```python
from build123d import *

# Parameters (mm, degrees)
F1_DEPTH = 200
F2_R     = 2
F3_DEPTH = 7.301
F6_DEPTH = 25
F9_DEPTH = 150


# Not quite as in the source:
# - a feature names something its author has since deleted; it is built from what else it names


with BuildPart() as f1:
    # F0 (on Front) → F1 (new body)
    with BuildSketch(Plane.XZ):
        with BuildLine():
            Line((7.0581561667, 0.685534298), (6.15, 1.65))
            ThreePointArc((6.15, 1.65), (5.5642135624, 3.0642135624), (4.15, 3.65))
            Line((4.15, 3.65), (-4.15, 3.65))
            ThreePointArc((-4.15, 3.65), (-5.5642135624, 3.0642135624), (-6.15, 1.65))
            Line((-6.15, 1.65), (-7.0581561667, 0.685534298))
            ThreePointArc((-7.0581561667, 0.685534298), (-7.3301158338, 0), (-7.0581561667, -0.685534298))
            Line((-7.0581561667, -0.685534298), (-6.15, -1.65))
            ThreePointArc((-6.15, -1.65), (-5.5642135624, -3.0642135624), (-4.15, -3.65))
            Line((-4.15, -3.65), (4.15, -3.65))
            ThreePointArc((4.15, -3.65), (5.5642135624, -3.0642135624), (6.15, -1.65))
            Line((6.15, -1.65), (7.0581561667, -0.685534298))
            ThreePointArc((7.0581561667, -0.685534298), (7.3301158338, 0), (7.0581561667, 0.685534298))
        make_face()
        with BuildLine():
            ThreePointArc((5.15, -1.65), (4.8571067812, -2.3571067812), (4.15, -2.65))
            Line((4.15, -2.65), (-4.15, -2.65))
            ThreePointArc((-4.15, -2.65), (-4.8571067812, -2.3571067812), (-5.15, -1.65))
            Line((-5.15, -1.65), (-5.15, 1.65))
            ThreePointArc((-5.15, 1.65), (-4.8571067812, 2.3571067812), (-4.15, 2.65))
            Line((-4.15, 2.65), (4.15, 2.65))
            ThreePointArc((4.15, 2.65), (4.8571067812, 2.3571067812), (5.15, 1.65))
            Line((5.15, 1.65), (5.15, -1.65))
        make_face(mode=Mode.SUBTRACT)
        with BuildLine():
            Line((-4.15, -2.65), (4.15, -2.65))
            ThreePointArc((4.15, -2.65), (4.8571067812, -2.3571067812), (5.15, -1.65))
            Line((5.15, -1.65), (5.15, 1.65))
            ThreePointArc((5.15, 1.65), (4.8571067812, 2.3571067812), (4.15, 2.65))
            Line((4.15, 2.65), (-4.15, 2.65))
            ThreePointArc((-4.15, 2.65), (-4.8571067812, 2.3571067812), (-5.15, 1.65))
            Line((-5.15, 1.65), (-5.15, -1.65))
            ThreePointArc((-5.15, -1.65), (-4.8571067812, -2.3571067812), (-4.15, -2.65))
        make_face()
    extrude(amount=F1_DEPTH)

    # F2 (on face) → F3 (cut, through all)
    with BuildSketch(Plane.XY.offset(3.65)):
        with Locations((0, -5)):
            Circle(F2_R)
    extrude(amount=-F3_DEPTH, mode=Mode.SUBTRACT)

    # F5 (on offset) → F6 (cut)
    with BuildSketch(Plane.XY.offset(4.6)):
        with BuildLine():
            Line((8, -3.7011680724), (8, 3.7011680724))
            Line((8, 3.7011680724), (-8, 3.7011680724))
            Line((-8, 3.7011680724), (-8, -3.7011680724))
            ThreePointArc((-8, -3.7011680724), (0, -0.1482238292), (8, -3.7011680724))
        make_face()
    extrude(amount=-F6_DEPTH, mode=Mode.SUBTRACT)

    # F8 (on offset) → F9 (cut)
    with BuildSketch(Plane.XZ.offset(200)):
        Polygon((-5.1262229681, -2.646596171), (0, -2.646596171), (5.1262229681, -2.646596171), (5.1262229681, -0.6600963534), (4.3867812492, 3.7468392402), (0, 3.7468392402), (-4.3867812492, 3.7468392402), (-5.1262229681, -0.6600963534), align=None)
    extrude(amount=-F9_DEPTH, mode=Mode.SUBTRACT)


solid = f1.part
```
Here's how the part is built. I have some questions about the finished solid (model axes, mm). A direction names the side the tool comes from. Coordinates: 2 decimals unless noted, no trailing zeros. Loops run counter-clockwise (first coordinate to the right, second up) from the corner with the lowest first, then second, coordinate; pieces in that order, holes last. Notation, with made-up numbers: (3.5, -30) - (20.5, -30) arc R25 cw to (20.5, -17) - close; hole circle Ø6 at (73.25, 76.25). An arc over 180 degrees is marked (long way). Return JSON: item names as keys, results as strings. Group by question number.
Item 1: If we section it at B-B on x = 0: Write out the boundary of the cut face in (y, z), and give its area (3 significant figures).
Item 2: We'd pull the mould along X, two halves only. Please class faces 1 (the face through (-1, -200, -3)), 2 (the face through (-4.76, -126.05, 1.52)), 3 (the face through (-0.11, -0.15, 0.05)): +X half, -X half, draft (parallel to the pull), parting line (faces both ways), or undercut.
Item 3: I need wall thicknesses on line 1 (Y direction, x = 0, z = 0.5); line 2 (Z direction, x = 0, y = -83); line 3 (X direction, y = -49, z = 2). Which ranges of each line are inside material? Lowest first, please. Write a range as from..to.
Item 4: If we section it at A-A on y = -5: Write out the boundary of the cut face in (x, z).
Item 5: Will these pins go through, and if not, where does the flat tip stop? P1, Ø2, axis at x = 4, y = -124, coming from the +Z side; P2, Ø2, axis at x = 1.5, z = -1, coming from the +Y side; P3, Ø2, axis at y = -59, z = -0.5, coming from the -X side; P4, Ø1, axis at y = -131, z = -1.5, coming from the +X side.
Item 6: If we section it at C-C on y = -55: Write out the boundary of the cut face in (x, z).
Item 7: On a 3-axis mill with a long thin cutter (end or side, diameter ignored), from which of +Z, -Z, +X, -X, +Y, -Y can I reach the whole of each face in a straight line? I mean faces 4 (the face through (0, -99, -3.65)), 5 (the face through (4.77, -126.05, 1.46)). Say none if no direction works.
Calculated:
{
 "1": {"outline": "(-200, -3.65) - (-7, -3.65) - (-7, 3.65) - (-50, 3.65) - (-50, -2.65) - (-200, -2.65) - close; (-3, -3.65) - (-0.15, -3.65) - (-0.15, 3.65) - (-3, 3.65) - close", "area": "485 mm^2"},
 "2": {"face 1": "draft", "face 2": "undercut", "face 3": "parting line"},
 "3": {"line 1": "y = -50..-7, -3..-0.15", "line 2": "z = -3.65..-2.65", "line 3": "x = -6.12..6.12"},
 "4": {"outline": "(-7.06, -0.69) - (-6.15, -1.65) arc R2 ccw to (-4.15, -3.65) - (-2, -3.65) - (-2, 3.65) - (-4.15, 3.65) arc R2 ccw to (-6.15, 1.65) - (-7.06, 0.69) arc R1 ccw to start; (2, -3.65) - (4.15, -3.65) arc R2 ccw to (6.15, -1.65) - (7.06, -0.69) arc R1 ccw to (7.06, 0.69) - (6.15, 1.65) arc R2 ccw to (4.15, 3.65) - (2, 3.65) - close"},
 "5": {"P1": "stops at z = 3.63", "P2": "stops at y = -0.16", "P3": "stops at x = -7.33", "P4": "stops at x = 6.76"},
 "6": {"outline": "(-7.06, -0.69) - (-6.15, -1.65) arc R2 ccw to (-4.15, -3.65) - (4.15, -3.65) arc R2 ccw to (6.15, -1.65) - (7.06, -0.69) arc R1 ccw to (7.06, 0.69) - (6.15, 1.65) arc R2 ccw to (4.41, 3.63) - (5.13, -0.66) - (5.13, -2.65) - (-5.13, -2.65) - (-5.13, -0.66) - (-4.41, 3.63) arc R2 ccw to (-6.15, 1.65) - (-7.06, 0.69) arc R1 ccw to start"},
 "7": {"face 4": "-Z, +X, -X, +Y, -Y", "face 5": "-Y"}
}
